For this review, take the finished solid that the model builds, in its own axes (mm). Face numbers are marked on the shaded views. A direction names the side the tool comes from. Round coordinates to 2 decimals unless told otherwise and drop trailing zeros. Loops run counter-clockwise (first coordinate to the right, second up) from the corner with the lowest first, then second, coordinate; pieces in that order, holes last.
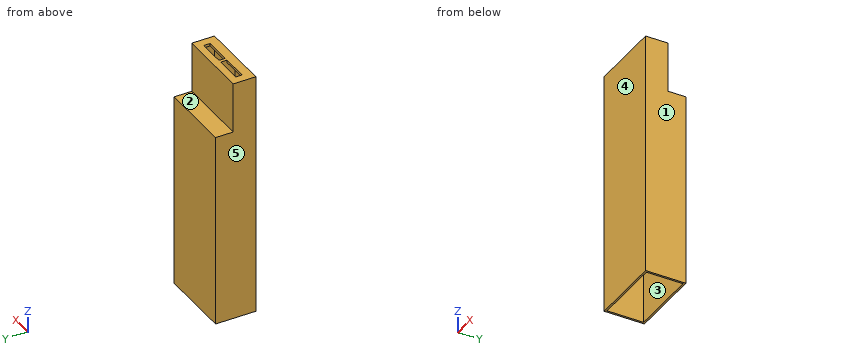
```python
from build123d import *

# Parameters (mm, degrees)
SKETCH1_W           = 58
SKETCH1_H           = 18
SKETCH1_W_2         = 21.15
SKETCH1_H_2         = 5
BOSS_EXTRUDE1_DEPTH = 40
SKETCH2_W           = 58
SKETCH2_H           = 32
BOSS_EXTRUDE2_DEPTH = 155
CUT_EXTRUDE1_START  = 2
SKETCH3_W           = 55
SKETCH3_H           = 16.5
CUT_EXTRUDE1_DEPTH  = 39
SKETCH4_W           = 2.5
SKETCH4_H           = 16.5
BOSS_EXTRUDE3_DEPTH = 20
FILLET1_R           = 1.25
SKETCH5_W           = 55
SKETCH5_H           = 29
CUT_EXTRUDE2_DEPTH  = 153.5
SKETCH6_W           = 55
SKETCH6_H           = 16.5
CUT_EXTRUDE3_DEPTH  = 153.5


with BuildPart() as part:
    # Sketch1 → Boss-Extrude1 (new body)
    with BuildSketch(Plane.XY):
        Rectangle(SKETCH1_W, SKETCH1_H)
        with Locations((-11.825, 0.7)):
            Rectangle(SKETCH1_W_2, SKETCH1_H_2, mode=Mode.SUBTRACT)
        with Locations((11.825, 0.7)):
            Rectangle(SKETCH1_W_2, SKETCH1_H_2, mode=Mode.SUBTRACT)
    extrude(amount=BOSS_EXTRUDE1_DEPTH)

    # Sketch2 → Boss-Extrude2 (add)
    with BuildSketch(Plane(origin=(0, 0, 0), x_dir=(-1, 0, 0), z_dir=(0, 0, -1))):
        with Locations((0, 7)):
            Rectangle(SKETCH2_W, SKETCH2_H)
    extrude(amount=BOSS_EXTRUDE2_DEPTH)

    # Sketch3 → Cut-Extrude1 (cut)
    with BuildSketch(Plane(origin=(0, 0, 40), x_dir=(-1, 0, 0), z_dir=(0, 0, -1)).offset(CUT_EXTRUDE1_START)):
        Rectangle(SKETCH3_W, SKETCH3_H)
    extrude(amount=CUT_EXTRUDE1_DEPTH, mode=Mode.SUBTRACT)

    # Sketch4 → Boss-Extrude3 (add)
    with BuildSketch(Plane(origin=(0, 0, 40), x_dir=(-1, 0, 0), z_dir=(0, 0, -1))):
        Rectangle(SKETCH4_W, SKETCH4_H)
    extrude(amount=BOSS_EXTRUDE3_DEPTH)

    # Fillet1
    fillet1_edges = [part.edges().sort_by_distance(p)[0] for p in [
        (1.25, 0, 20),
        (-1.25, 0, 20),
    ]]
    fillet(fillet1_edges, radius=FILLET1_R - 0.0001)  # a hair under: the kernel refuses the full size

    # Sketch5 → Cut-Extrude2 (cut)
    with BuildSketch(Plane(origin=(0, 0, -155), x_dir=(-1, 0, 0), z_dir=(0, 0, -1))):
        with Locations((0, 7)):
            Rectangle(SKETCH5_W, SKETCH5_H)
    extrude(amount=-CUT_EXTRUDE2_DEPTH, mode=Mode.SUBTRACT)

    # Sketch6 → Cut-Extrude3 (cut)
    with BuildSketch(Plane.XY.offset(-1)):
        Rectangle(SKETCH6_W, SKETCH6_H)
    extrude(amount=-CUT_EXTRUDE3_DEPTH, mode=Mode.SUBTRACT)


solid = part.part
```
(1) For L1, parallel to Y at x = 12, z = -13.5; L2, parallel to X at y = 6.5, z = -47; L3, parallel to Y at x = 9, z = 31.5, list the stretches that pass through material, from the lowest coordinate up.
(2) Add section C-C (z = 18). Give the boundary of the cut face in (x, y), plus the area to 4 significant figures.
(3) Add section A-A (x = 19.5). Give the boundary of the cut face in (y, z), plus the area to 3 significant figures.
(4) The part is to be moulded in two halves that separate along Y. For the marked faces 3, 4 and 5, say which applies: pulls with the +Y half, pulls with the -Y half, needs draft (parallel to the pull), parting line crosses it, or undercut.
(5) Add section D-D (y = 12.5). Give the boundary of the cut face in (x, z).
(6) Add section B-B (y = 0). Give the number of separate pieces and of enclosed holes in the cut face, plus the area to 3 significant figures.
(7) Insertion check: pin 1 Ø0.6 at (x, z) = (-10, 39) entering from +Y; pin 2 Ø1.5 at (x, y) = (-11, 13.5) entering from -Z; pin 3 Ø8 at (x, y) = (-19, 3.5) entering from -Z; pin 4 Ø10 at (x, y) = (12.5, 11.5) entering from +Z. Each pin has a flat end and moves straight along its axis. Give the tip position at first contact, or say it passes through.
(8) For the marked faces 1 and 2, list the 3-axis set-ups (+Z, -Z, +X, -X, +Y, -Y) from which the entire face can be reached by the end or side of a thin tool; tool diameter is ignored.
Outcome:
1. L1: y = -9 to -8.25, 21.5 to 23
1. L2: x = -29 to -27.5, 27.5 to 29
1. L3: y = -9 to -8.25, 8.25 to 9
2. outline: (-29, -9) - (29, -9) - (29, 9) - (-29, 9) - close; hole (-27.5, -8.25) - (27.5, -8.25) - (27.5, 8.25) - (-27.5, 8.25) - close
2. area: 136.5 mm2
3. outline: (-9, -155) - (-7.5, -155) - (-7.5, -154.5) - (-8.25, -154.5) - (-8.25, 38) - (-1.8, 38) - (-1.8, 40) - (-9, 40) - close; (3.2, 38) - (8.25, 38) - (8.25, -1.5) - (21.5, -1.5) - (21.5, -155) - (23, -155) - (23, 0) - (9, 0) - (9, 40) - (3.2, 40) - close
3. area: 452 mm2
4. face 3: undercut
4. face 4: pulls with the -Y half
4. face 5: needs draft
5. outline: (-29, -155) - (-27.5, -155) - (-27.5, -1.5) - (27.5, -1.5) - (27.5, -155) - (29, -155) - (29, 0) - (-29, 0) - close
6. separate pieces: 3
6. enclosed holes: 0
6. area: 655 mm2
7. pin 1: stops at y = 9
7. pin 2: stops at z = -1.5
7. pin 3: stops at z = 38
7. pin 4: stops at z = 40
8. face 1: +Z, -Z, +X, +Y, -Y
8. face 2: +Z, +X, -X, +Y
